Design review of the part built by this model. Coordinates are the model's own, in mm. Face numbers are marked on the shaded views. A direction names the side the tool comes from. Coordinates: 2 decimals unless noted, no trailing zeros. Order: outer loops, then holes, each group sorted by start corner. A loop starts at its lowest first (then second) coordinate and runs counter-clockwise, first axis right, second up. Notation, with made-up numbers: M -17.75,1 L 11.25,1 A25 cw 11.25,26 Z; hole C 74,-31.75 d9. An arc over 180 degrees is marked long. Answer as a JSON object with one key per item and string values.
from build123d import *

# Parameters (mm, degrees)
SKETCH1_R           = 10
BOSS_EXTRUDE1_DEPTH = 10
CUT_EXTRUDE1_REACH  = 19.321
SKETCH2_R           = 1.7
SKETCH3_R           = 3.5
CUT_EXTRUDE2_DEPTH  = 3.2
CHAMFER1_SIZE       = 0.4
CHAMFER2_SIZE       = 0.4


with BuildPart() as part:
    # Sketch1 → Boss-Extrude1 (new body)
    with BuildSketch(Plane.XY):
        Circle(SKETCH1_R)
    extrude(amount=BOSS_EXTRUDE1_DEPTH)

    # Sketch2 → Cut-Extrude1 (cut, up to next)
    with BuildSketch(Plane.XY.offset(10), mode=Mode.PRIVATE) as cut_extrude1_sk1:
        Circle(SKETCH2_R)
    cut_extrude1_tool1 = extrude(cut_extrude1_sk1.sketch, amount=-CUT_EXTRUDE1_REACH, mode=Mode.PRIVATE) & part.part
    add(cut_extrude1_tool1.solids().sort_by_distance((0, 0, 10))[0], mode=Mode.SUBTRACT)

    # Sketch3 → Cut-Extrude2 (cut)
    with BuildSketch(Plane.XY.offset(10)):
        Circle(SKETCH3_R)
    cut_extrude2 = extrude(amount=-CUT_EXTRUDE2_DEPTH, mode=Mode.SUBTRACT)

    # Mirror1: Cut-Extrude2 across plane
    add(cut_extrude2.mirror(Plane.XY.offset(5)), mode=Mode.SUBTRACT)

    # Sketch4 → Cut-Revolve1 (revolve, cut)
    with BuildSketch(Plane(origin=(0, 0, 0), x_dir=(1, 0, 0), z_dir=(0, 1, 0)), mode=Mode.PRIVATE) as cut_revolve1_sk:
        with BuildLine():
            Line((10, -10), (10, 0))
            ThreePointArc((10, 0), (8.566018868, -5), (10, -10))
        make_face()
    revolve(cut_revolve1_sk.sketch.rotate(Axis((0, 0, 3.2), (0, 0, 1)), 180), axis=Axis((0, 0, 3.2), (0, 0, 1)), mode=Mode.SUBTRACT)

    # Chamfer1
    # the kernel refuses this chamfer: 0.4, 0.290276343 mm, written as the material it takes off along each edge
    with BuildSketch(Plane(origin=(0, 0, 10), x_dir=(1, 0, 0), z_dir=(0, -1, 0))) as chamfer1_piece_1:
        Polygon((3.5, -CHAMFER1_SIZE), (3.5 + CHAMFER1_SIZE, 0), (3.5, 0), align=None)
    revolve(axis=Axis((0, 0, 10), (0, 0, 1)), mode=Mode.SUBTRACT)
    with BuildSketch(Plane(origin=(0, 0, 0), x_dir=(1, 0, 0), z_dir=(0, -1, 0))) as chamfer1_piece_2:
        Polygon((3.5 + CHAMFER1_SIZE, 0), (3.5, CHAMFER1_SIZE), (3.5, 0), align=None)
    revolve(axis=Axis((0, 0, 0), (0, 0, 1)), mode=Mode.SUBTRACT)
    with BuildSketch(Plane(origin=(0, 0, 10), x_dir=(-1, 0, 0), z_dir=(0, -1, 0))) as chamfer1_piece_3:
        with BuildLine():
            Line((10 - CHAMFER1_SIZE, 0), (9.849418631, 0.249418631))
            ThreePointArc((9.849418631, 0.249418631), (9.922753807, 0.125772477), (10, 0))
            Line((10, 0), (10 - CHAMFER1_SIZE, 0))
        make_face()
    revolve(axis=Axis((0, 0, 10), (0, 0, -1)), mode=Mode.SUBTRACT)

    # Chamfer2
    # the kernel refuses this chamfer: 0.4, 0.290276343 mm, written as the material it takes off along each edge
    with BuildSketch(Plane(origin=(0, 0, 0), x_dir=(-1, 0, 0), z_dir=(0, -1, 0))) as chamfer2_piece_1:
        with BuildLine():
            Line((10 - CHAMFER2_SIZE, 0), (9.849418631, -0.249418631))
            ThreePointArc((9.849418631, -0.249418631), (9.922753807, -0.125772477), (10, 0))
            Line((10, 0), (10 - CHAMFER2_SIZE, 0))
        make_face()
    revolve(axis=Axis((0, 0, 0), (0, 0, -1)), mode=Mode.SUBTRACT)


solid = part.part
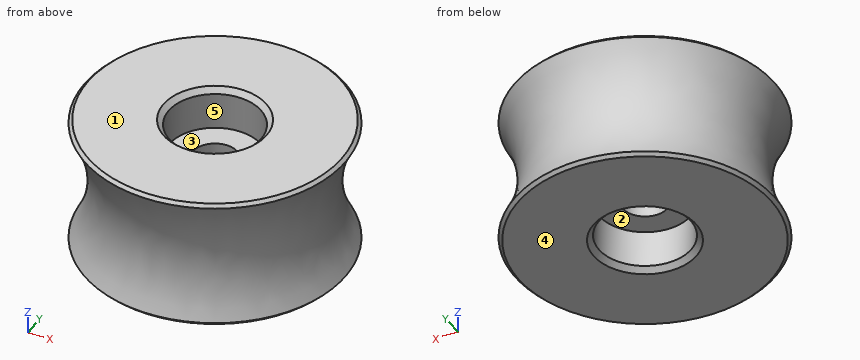
1) Mouldability with a two-part tool opening along Y and no side actions: class the marked faces 4 and 5 as released by +Y, released by -Y, zero draft, split by the parting line, or undercut.
Taken from the geometry:
{"face 4": "zero draft", "face 5": "undercut"}
2) Add section D-D (z = 4). State the section outline as (x, y) points.
Taken from the geometry:
{"outline": "C 0,0 d17.24; hole C 0,0 d3.4"}
3) Add section A-A (y = 0). State the section outline as (x, z) points.
Taken from the geometry:
{"outline": "M -9.85,0.25 L -9.6,0 L -3.9,0 L -3.5,0.4 L -3.5,3.2 L -1.7,3.2 L -1.7,6.8 L -3.5,6.8 L -3.5,9.6 L -3.9,10 L -9.6,10 L -9.85,9.75 A9.43 cw Z; M 1.7,3.2 L 3.5,3.2 L 3.5,0.4 L 3.9,0 L 9.6,0 L 9.85,0.25 A9.43 cw 9.85,9.75 L 9.6,10 L 3.9,10 L 3.5,9.6 L 3.5,6.8 L 1.7,6.8 Z"}
4) To check wall thickness, follow L1, parallel to Z at x = 1, y = 2.5; L2, parallel to X at y = 1.5, z = 8.5; L3, parallel to Y at x = 0, z = 1.65. State the ranges of each line that lie inside material, in increasing order.
Taken from the geometry:
{"L1": "z = 3.2 to 6.8", "L2": "x = -9.12 to -3.16, 3.16 to 9.12", "L3": "y = -9.18 to -3.5, 3.5 to 9.18"}
5) Insertion check: pin 1 Ø4 at (x, y) = (0, 0) entering from +Z; pin 2 Ø1 at (x, z) = (-5.5, 8) entering from -Y; pin 3 Ø3.5 at (x, y) = (1, 0) entering from -Z. Each pin has a flat end and moves straight along its axis. Give the tip position at first contact, or say it passes through.
Taken from the geometry:
{"pin 1": "stops at z = 6.8", "pin 2": "stops at y = -7.61", "pin 3": "stops at z = 3.2"}
6) Tool access review of the marked faces 1, 2 and 3: name each direction out of +Z, -Z, +X, -X, +Y, -Y from which nothing blocks a thin tool from reaching the whole face with its end or side.
Taken from the geometry:
{"face 1": "+Z, +X, -X, +Y, -Y", "face 2": "-Z", "face 3": "+Z"}
7) Add section C-C (z = 8.5). State the section outline as (x, y) points, and give its area (3 significant figures).
Taken from the geometry:
{"outline": "C 0,0 d18.48; hole C 0,0 d7", "area": "230 mm2"}
